Geometry: final body of the model. Coordinates: model frame, mm. Give positions to 0.01 mm unless a question says otherwise; leave off trailing zeros. Order: outer loops, then holes, each group sorted by start corner. A loop starts at its lowest first (then second) coordinate and runs counter-clockwise, first axis right, second up. Notation, with made-up numbers: (40, 78.5) -> (56, 78.5) arc R22 cw to (56, 105.5) -> close; hole circle Ø5 at (9.25, 75). An arc over 180 degrees is marked (long way). Write item = value, one per line.
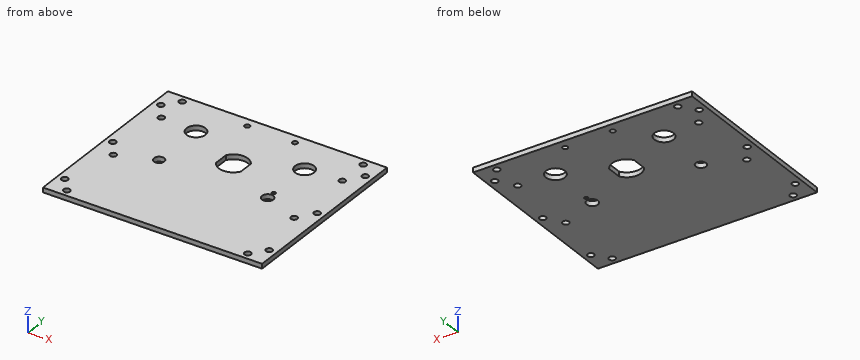
```python
from build123d import *

# Parameters (mm, degrees)
SKETCH1_W             = 146.05
SKETCH1_H             = 123.825
BOSS_EXTRUDE1_DEPTH   = 3.175
F_6_CLEARANCE_HOLE1_D = 4.3053
SKETCH4_R             = 6.35
SKETCH4_R_2           = 3.7703125
SKETCH4_R_3           = 3.429
SKETCH4_R_4           = 1.190625
CUT_EXTRUDE1_DEPTH    = 4.175
F_4_CLEARANCE_HOLE1_D = 3.4544


with BuildPart() as part:
    # Sketch1 → Boss-Extrude1 (new body)
    with BuildSketch(Plane.XY):
        with Locations((-73.025, 61.9125)):
            Rectangle(SKETCH1_W, SKETCH1_H)
    extrude(amount=-BOSS_EXTRUDE1_DEPTH)

    # #6 Clearance Hole1 (through all)
    with Locations(Plane(origin=(0, 0, -3.175), x_dir=(-1, 0, 0), z_dir=(0, 0, -1))):
        with Locations((12.7, 119.0625), (133.35, 119.0625), (141.1605, 109.5375), (133.35, 98.425), (141.1605, 61.9125), (133.35, 50.673), (133.35, 4.7625), (12.7, 4.7625), (12.7, 50.673), (12.7, 98.425), (4.8895, 109.5375), (141.1605, 14.2875), (4.8895, 14.2875), (4.8895, 61.9125)):
            Hole(F_6_CLEARANCE_HOLE1_D / 2)

    # Sketch4 → Cut-Extrude1 (cut, through all)
    with BuildSketch(Plane(origin=(0, 0, -3.175), x_dir=(-1, 0, 0), z_dir=(0, 0, -1))):
        with Locations((36.83, 96.901)):
            Circle(SKETCH4_R)
        with Locations((36.83, 60.325)):
            Circle(SKETCH4_R_2)
        with Locations((109.22, 60.325)):
            Circle(SKETCH4_R_3)
        with Locations((109.22, 96.901)):
            Circle(SKETCH4_R)
        with Locations((36.830000026, 66.325)):
            Circle(SKETCH4_R_4)
        with BuildLine():
            Line((81.3435, 85.032269324), (81.3435, 75.241730676))
            ThreePointArc((81.3435, 75.241730676), (73.025, 70.485), (64.7065, 75.241730676))
            Line((64.7065, 75.241730676), (64.7065, 85.032269324))
            ThreePointArc((64.7065, 85.032269324), (73.025, 89.789), (81.3435, 85.032269324))
        make_face()
    extrude(amount=-CUT_EXTRUDE1_DEPTH, mode=Mode.SUBTRACT)

    # #4 Clearance Hole1 (through all)
    with Locations(Plane.XY):
        with Locations((-88.9, 117.475), (-57.15, 117.475)):
            Hole(F_4_CLEARANCE_HOLE1_D / 2)


solid = part.part
```
1) Section query C-C (z = -1.9). Count the separate pieces of the cut face and the enclosed holes in it, plus the area to 3 significant figures.
Check sheet entries:
separate_pieces = 1
enclosed_holes = 22
area = 17,200 mm²
2) Section query A-A (x = -12.7). Output: boundary loops of the cut face in (y, z) (3 decimals).
Check sheet entries:
outline = (0, -3.175) -> (2.61, -3.175) -> (2.61, 0) -> (0, 0) -> close; (6.915, -3.175) -> (48.52, -3.175) -> (48.52, 0) -> (6.915, 0) -> close; (52.826, -3.175) -> (96.272, -3.175) -> (96.272, 0) -> (52.826, 0) -> close; (100.578, -3.175) -> (116.91, -3.175) -> (116.91, 0) -> (100.578, 0) -> close; (121.215, -3.175) -> (123.825, -3.175) -> (123.825, 0) -> (121.215, 0) -> close
3) Section query B-B (x = -109.22). Output: boundary loops of the cut face in (y, z) (3 decimals), plus the area to 3 significant figures.
Check sheet entries:
outline = (0, -3.175) -> (56.896, -3.175) -> (56.896, 0) -> (0, 0) -> close; (63.754, -3.175) -> (90.551, -3.175) -> (90.551, 0) -> (63.754, 0) -> close; (103.251, -3.175) -> (123.825, -3.175) -> (123.825, 0) -> (103.251, 0) -> close
area = 331 mm²
4) First-contact query: P1, Ø5, axis at x = -141.16, y = 14.29, coming from the +Z side. Flat tip, straight axial feed; report the tip coordinate or a pass-through.
Check sheet entries:
P1 = 0
5) Line query: line 1 (Y direction, x = -12.7, z = -1.05) (3 decimals); line 2 (Y direction, x = -109.22, z = -1.4) (3 decimals); line 3 (X direction, y = 60, z = -0.55). Output: solid intervals per line, ascending. Write a range as from..to.
Check sheet entries:
line_1 = 0..2.61, 6.915..48.52, 52.826..96.272, 100.578..116.91, 121.215..123.825
line_2 = 0..56.896, 63.754..90.551, 103.251..123.825
line_3 = -146.05..-142.15, -140.17..-112.63, -105.81..-40.59, -33.07..-5.88, -3.9..0
